from build123d import *

# Parameters (mm, degrees)
F0_W     = 31.75
F0_H     = 9.652
F1_DEPTH = 15.7988
F2_R     = 2.4384
F3_DEPTH = 1.778
F4_W     = 29.3116
F4_H     = 13.3604
F4_R     = 3.2512
F4_R_2   = 2.4384
F5_DEPTH = 8.4328


with BuildPart() as f1:
    # F0 (on Front) → F1 (new body)
    with BuildSketch(Plane.XZ):
        with Locations((-15.875, -4.826)):
            Rectangle(F0_W, F0_H)
    extrude(amount=F1_DEPTH)

    # F2 (on face) → F3 (join)
    with BuildSketch(Plane.XY):
        with Locations((-27.8384, -3.9116)):
            Circle(F2_R)
        with Locations((-19.7612, -3.9116)):
            Circle(F2_R)
        with Locations((-11.684, -3.9116)):
            Circle(F2_R)
        with Locations((-3.6068, -3.9116)):
            Circle(F2_R)
        with Locations((-3.6068, -12.0142)):
            Circle(F2_R)
        with Locations((-11.684, -12.0142)):
            Circle(F2_R)
        with Locations((-19.7612, -12.0142)):
            Circle(F2_R)
        with Locations((-27.8384, -12.0142)):
            Circle(F2_R)
    extrude(amount=F3_DEPTH)

    # F4 (on face) → F5 (cut)
    with BuildSketch(Plane(origin=(0, 0, -9.652), x_dir=(1, 0, 0), z_dir=(0, 0, -1))):
        with Locations((-15.875, 7.8994)):
            Rectangle(F4_W, F4_H)
        with Locations((-23.8506, 7.8994)):
            Circle(F4_R, mode=Mode.SUBTRACT)
        with Locations((-15.8496, 7.8994)):
            Circle(F4_R, mode=Mode.SUBTRACT)
        with Locations((-7.8486, 7.8994)):
            Circle(F4_R, mode=Mode.SUBTRACT)
        with Locations((-23.8506, 7.8994)):
            Circle(F4_R_2)
        with Locations((-15.8496, 7.8994)):
            Circle(F4_R_2)
        with Locations((-7.8486, 7.8994)):
            Circle(F4_R_2)
    extrude(amount=-F5_DEPTH, mode=Mode.SUBTRACT)


solid = f1.part
Verification items for the finished model (mm, model axes). A direction names the side the tool comes from. Coordinates: 2 decimals unless noted, no trailing zeros. Order: outer loops, then holes, each group sorted by start corner. A loop starts at its lowest first (then second) coordinate and runs counter-clockwise, first axis right, second up. Notation, with made-up numbers: M -11.5,37 L 5.5,37 A5 ccw 5.5,41 Z; hole C -24.5,-27 d4. An arc over 180 degrees is marked long. Return JSON: item names as keys, results as strings.
1) Gauge pin test, flat ends, axial feed: pin 1 (5.5 mm diameter, centred on x = -23.85, y = -7.9, fed in from +Z); pin 2 (1 mm diameter, centred on x = -3.5, y = -6.5, fed in from -Z). Record the tip position at first contact, or that the pin passes through.
Answer list:
{"pin 1": "z = 0", "pin 2": "z = -1.22"}
2) Cross-section at D-D, the plane y = -13.75. Record the boundary of the cut face in (x, z), and give its area (3 significant figures).
Answer list:
{"outline": "M -31.75,-9.65 L -30.53,-9.65 L -30.53,-1.22 L -1.22,-1.22 L -1.22,-9.65 L 0,-9.65 L 0,0 L -1.89,0 L -1.89,1.78 L -5.32,1.78 L -5.32,0 L -9.97,0 L -9.97,1.78 L -13.4,1.78 L -13.4,0 L -18.05,0 L -18.05,1.78 L -21.47,1.78 L -21.47,0 L -26.13,0 L -26.13,1.78 L -29.55,1.78 L -29.55,0 L -31.75,0 Z", "area": "83.6 mm2"}
3) Cross-section at C-C, the plane x = -15. Record the boundary of the cut face in (y, z) (3 decimals).
Answer list:
{"outline": "M -15.799,-9.652 L -14.58,-9.652 L -14.58,-1.219 L -11.038,-1.219 L -11.038,-9.652 L -10.185,-9.652 L -10.185,-1.219 L -5.614,-1.219 L -5.614,-9.652 L -4.761,-9.652 L -4.761,-1.219 L -1.219,-1.219 L -1.219,-9.652 L 0,-9.652 L 0,0 L -15.799,0 Z"}
4) Cross-section at A-A, the plane z = -8. Record the boundary of the cut face in (x, y).
Answer list:
{"outline": "M -31.75,-15.8 L 0,-15.8 L 0,0 L -31.75,0 Z; C -23.85,-7.9 d6.5; C -15.85,-7.9 d6.5; C -7.85,-7.9 d6.5; hole M -30.53,-14.58 L -1.22,-14.58 L -1.22,-1.22 L -30.53,-1.22 Z; hole C -23.85,-7.9 d4.88; hole C -15.85,-7.9 d4.88; hole C -7.85,-7.9 d4.88"}
5) Thickness scan on L1, parallel to X at y = -1.25, z = -1.75; L2, parallel to X at y = -2.5, z = 1; L3, parallel to Y at x = -28, z = -3.75. Record the ranges inside material, lowest first. Write a range as [from, to].
Answer list:
{"L1": "[-31.75, -30.53], [-1.22, 0]", "L2": "[-29.83, -25.85], [-21.75, -17.77], [-13.67, -9.7], [-5.6, -1.62]", "L3": "[-15.8, -14.58], [-1.22, 0]"}
6) Release check for a two-part mould opening along X. For faces 4 (the cylindrical face through (-14.12, -3.8, 0.88)), 5 (the flat face through (-23, -5, -9.652)), 6 (the flat face through (-31.75, -8, -5)) record: +X half, -X half, draft (parallel to the pull), parting line (faces both ways), or undercut.
Answer list:
{"face 4": "undercut", "face 5": "draft", "face 6": "-X half"}
7) Cross-section at B-B, the plane z = 0.5. Record the boundary of the cut face in (x, y).
Answer list:
{"outline": "C -27.84,-12.01 d4.88; C -27.84,-3.91 d4.88; C -19.76,-12.01 d4.88; C -19.76,-3.91 d4.88; C -11.68,-12.01 d4.88; C -11.68,-3.91 d4.88; C -3.61,-12.01 d4.88; C -3.61,-3.91 d4.88"}
8) Access from +Z, -Z, +X, -X, +Y, -Y to the whole of each face (thin tool, end or side, straight path). Record for faces 1 (the flat face through (-19.3, -8, -1.219)), 2 (the cylindrical face through (-12.213, -14.395, 0.877)), 3 (the flat face through (-20, -12, 1.778)).
Answer list:
{"face 1": "-Z", "face 2": "+Z", "face 3": "+Z, +X, -X, +Y, -Y"}
